Model file for the job. Use its own axes, mm. Round coordinates to 2 decimals unless told otherwise and drop trailing zeros. Order: outer loops, then holes, each group sorted by start corner. A loop starts at its lowest first (then second) coordinate and runs counter-clockwise, first axis right, second up. Notation, with made-up numbers: (75.25, -11) - (125.25, -11) arc R8 cw to (125.25, -2) - close; hole circle Ø10 at (3, 44). An arc over 180 degrees is marked (long way). Use one line per item in the form item = value.
from build123d import *

# Parameters (mm, degrees)
F7_R     = 37.5
F7_R_2   = 32.5
F8_DEPTH = 25


with BuildPart() as f2:
    # F1 (on offset) → F2 section 0
    with BuildSketch(Plane.XZ.offset(40), mode=Mode.PRIVATE) as f2_s0:
        Polygon((-7.2168783649, -12.5), (7.2168783649, -12.5), (14.4337567297, 0), (7.2168783649, 12.5), (-7.2168783649, 12.5), (-14.4337567297, 0), align=None)
    loft([Vertex(0, 0, 0), f2_s0.sketch])

    # F4 (on offset) → F6 section 0
    with BuildSketch(Plane.XZ.offset(40)):
        Polygon((-5.4848275573, -9.5), (5.4848275573, -9.5), (10.9696551146, 0), (5.4848275573, 9.5), (-5.4848275573, 9.5), (-10.9696551146, 0), align=None)
    # F5 (on offset) → F6 section 1
    with BuildSketch(Plane.XZ.offset(0.1)):
        Polygon((0.0180421959, 0.03125), (-0.0180421959, 0.03125), (-0.0360843918, 0), (-0.0180421959, -0.03125), (0.0180421959, -0.03125), (0.0360843918, 0), align=None)
    loft(mode=Mode.SUBTRACT)

    # F7 (on Top) → F8 (intersect, symmetric)
    with BuildSketch(Plane.XY):
        Circle(F7_R)
        Circle(F7_R_2, mode=Mode.SUBTRACT)
    extrude(amount=F8_DEPTH, both=True, mode=Mode.INTERSECT)


solid = f2.part
(1) Probe probe 1 along Z at (x, y) = (6, -33.5); probe 2 along Z at (x, y) = (9.25, -35.25); probe 3 along X at (y, z) = (-32.5, 5). List the from-to ranges inside material, lowest first. Write a range as [from, to].
Report:
probe_1 = [-10.47, -5.52], [5.52, 10.47]
probe_2 = [-6.01, -0.72], [0.72, 6.01]
probe_3 = [-8.84, -6.03], [6.03, 8.84]
(2) Slice it at A-A on z = -9.5. Give the cut face in (x, y).
Report:
outline = (-7.75, -36.69) arc R37.5 ccw to (7.75, -36.69) - (6.04, -31.93) arc R32.5 cw to (-6.04, -31.93) - close
(3) Pin check, flat tips, straight feed: pin 1 (1.5 mm diameter, centred on x = -10, z = -5.5, fed in from -Y); pin 2 (2 mm diameter, centred on x = -9, y = -36, fed in from +Z); pin 3 (2 mm diameter, centred on y = -35, z = -4, fed in from -X). Stop position of each tip, or through.
Report:
pin_1 = -36.34
pin_2 = 8.75
pin_3 = -11
(4) Pull direction X, two halves, no side cores. Call faces 1 (the face through (-9.023, -33.782, 5.485)), 2 (the face through (-0.09, -34.78, -10.87)), 3 (the face through (6.57, -31.83, 4.48)), 4 (the face through (7.582, -36.725, -5.17)): released by +X, released by -X, zero draft, split by the parting line, or undercut.
Report:
face_1 = released by -X
face_2 = zero draft
face_3 = undercut
face_4 = split by the parting line
